Design review of the part shown in the three views and the two pictorial views. Dimensions are in mm from the part's minimum x, y and z. Give positions to 0.01 mm unless a question says otherwise; leave off trailing zeros. Loops run counter-clockwise (first coordinate to the right, second up) from the corner with the lowest first, then second, coordinate; pieces in that order, holes last. Notation, with made-up numbers: (-38, 55) -> (-13, 55) arc R24 ccw to (-13, 79) -> close; hole circle Ø10 at (-18, 26.25). An arc over 180 degrees is marked (long way). Use CSV: the item, a comma, the result in double quotes. Start each with the question number.
Item 1: We need section D-D (y = 86.5). State the section outline as (x, z) points.
Item 2: We need section A-A (z = 3). State the section outline as (x, y) points (1 decimal).
Item 3: We need section B-B (y = 101). State the section outline as (x, z) points.
Item 4: We need section C-C (x = 20). State the section outline as (y, z) points (1 decimal), plus the area to 3 significant figures.
Item 5: The part is to be moulded in two halves that separate along X. For the marked faces 1, 2, 3 and 4, say which applies: +X half, -X half, draft (parallel to the pull), parting line (faces both ways), or undercut.
Item 6: Wall thickness on line 1 along Y through (x, z) = (76, 8) (1 decimal); line 2 along X through (y, z) = (101.5, 5.25) (1 decimal); line 3 along Y through (x, z) = (21.5, 0.75): over which ranges is each line inside the solid? List them lowest first. Write a range as from..to.
Item 7: Clearance check with flat-ended pins moving along their axes: pin 1 (2 mm diameter, centred on x = 18, z = 5.5, fed in from +Y); pin 2 (1 mm diameter, centred on y = 101.5, z = 9, fed in from -X); pin 3 (3 mm diameter, centred on y = 86, z = 2.5, fed in from +X) (1 decimal). State where each tip first meets the part, or that it passes through.
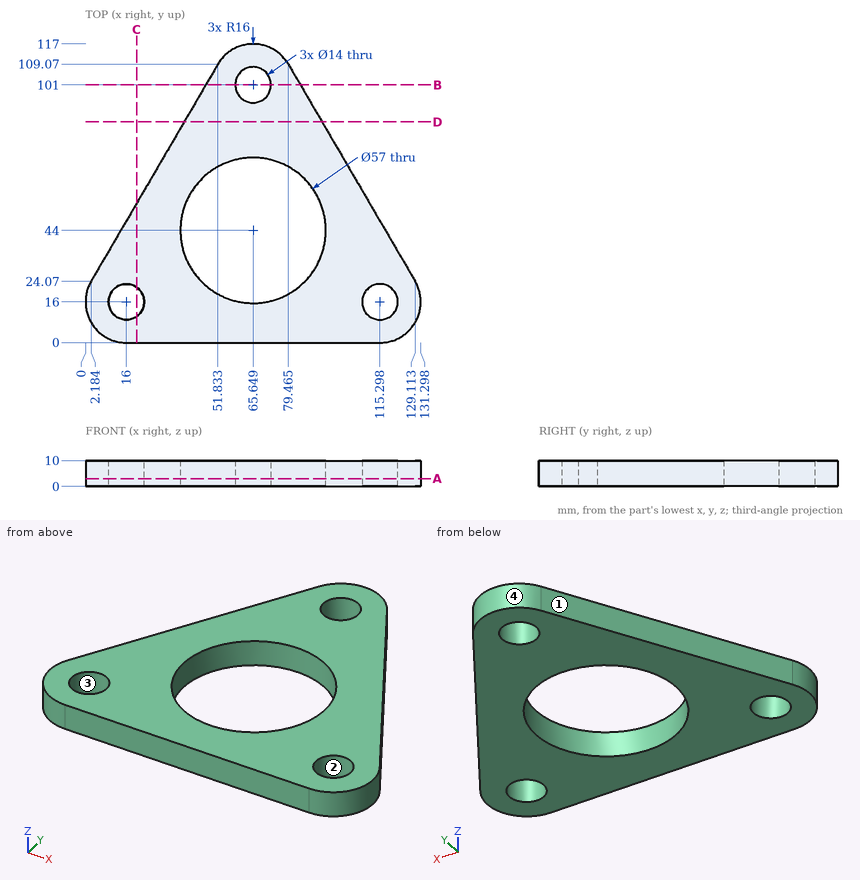
Results found:
1,outline,"(38.65, 0) -> (92.65, 0) -> (92.65, 10) -> (38.65, 10) -> close"
2,outline,"(2.2, 24.1) arc R16 ccw to (16, 0) -> (115.3, 0) arc R16 ccw to (129.1, 24.1) -> (79.5, 109.1) arc R16 ccw to (51.8, 109.1) -> close; hole circle Ø14 at (16, 16); hole circle Ø57 at (65.6, 44); hole circle Ø14 at (65.6, 101); hole circle Ø14 at (115.3, 16)"
3,outline,"(47.12, 0) -> (58.65, 0) -> (58.65, 10) -> (47.12, 10) -> close; (72.65, 0) -> (84.18, 0) -> (84.18, 10) -> (72.65, 10) -> close"
4,outline,"(0, 0) -> (10.3, 0) -> (10.3, 10) -> (0, 10) -> close; (21.7, 0) -> (54.6, 0) -> (54.6, 10) -> (21.7, 10) -> close"
4,area,"431 mm²"
5,face 1,"-X half"
5,face 2,"undercut"
5,face 3,"undercut"
5,face 4,"parting line"
6,line 1,"0..17.4, 70.6..113.2"
6,line 2,"47.4..58.7, 72.6..83.9"
6,line 3,"0..11.67, 20.33..57.14"
7,pin 1,"y = 52.86"
7,pin 2,"x = 47.12"
7,pin 3,"x = 93.8"
